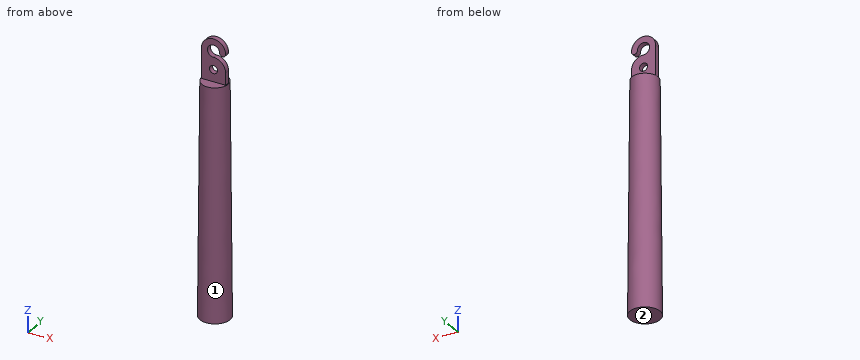
from build123d import *

# Parameters (mm, degrees)
F0_R     = 2
F1_DEPTH = 1.25


with BuildPart() as f1:
    # F0 (on Front) → F1 (new body, symmetric)
    with BuildSketch(Plane.XZ):
        with BuildLine():
            Line((-6, 15), (-6, 0))
            Line((-6, 0), (6, 0))
            Line((6, 0), (6, 6))
            ThreePointArc((6, 6), (4.242641, 10.242641), (0, 12))
            ThreePointArc((0, 12), (-2.12132, 17.12132), (3, 15))
            ThreePointArc((3, 15), (4.5, 13.5), (6, 15))
            ThreePointArc((6, 15), (0, 21), (-6, 15))
        make_face()
        with Locations((0, 6)):
            Circle(F0_R, mode=Mode.SUBTRACT)
    extrude(amount=F1_DEPTH, both=True)

    # F2 (on Right) → F3 (revolve)
    with BuildSketch(Plane.YZ):
        Polygon((0, -115), (0, 0), (-6.5, 0), (-7.5, -115), align=None)
    revolve(axis=Axis((0, 0, -57.5), (0, 0, -1)))


solid = f1.part
Check sheet for the modelled part. Datum: model origin and axes. Units: mm. Face numbers are marked on the shaded views. A direction names the side the tool comes from. Round coordinates to 2 decimals unless told otherwise and drop trailing zeros. Order: outer loops, then holes, each group sorted by start corner. A loop starts at its lowest first (then second) coordinate and runs counter-clockwise, first axis right, second up.
(1) Access from +Z, -Z, +X, -X, +Y, -Y to the whole of each face (thin tool, end or side, straight path). Record for the marked faces 1 and 2.
(2) Cross-section at B-B, the plane z = -93. Enter the section's corners in (x, y), and give its area (3 significant figures).
(3) Go/stop test with flat-tipped pins: P1, Ø8, axis at y = -6, z = -15.5, coming from the -X side; P2, Ø2, axis at y = 0.5, z = 7.5, coming from the -X side; P3, Ø7, axis at x = 0, z = 15, coming from the -Y side. Record where each tip stops, or that it passes through.
(4) Cross-section at A-A, the plane z = 1.5. Enter the section's corners in (x, y), and give its area (3 significant figures).
(5) Scan lines: probe 1 along Z at (x, y) = (0, 0.65); probe 2 along X at (y, z) = (-0.1, 15); probe 3 along Z at (x, y) = (-0.5, 1). Record each from-to range of solid material in increasing order.
Check sheet entries:
1. face 1: +Z
1. face 2: -Z, +X, -X, +Y, -Y
2. outline: circle Ø14.62 at (0, 0)
2. area: 168 mm2
3. P1: stops at x = -6.33
3. P2: stops at x = -6
3. P3: stops at y = -1.25
4. outline: (-6, -1.25) - (6, -1.25) - (6, 1.25) - (-6, 1.25) - close
4. area: 30.0 mm2
5. probe 1: z = -115 to 4, 8 to 12, 18 to 21
5. probe 2: x = -6 to -3, 3 to 6
5. probe 3: z = -115 to 4.06, 7.94 to 12.04, 17.96 to 20.98
